from build123d import *

# Parameters (mm, degrees)
F1_DEPTH = 25
F2_R     = 3.99999


# Not quite as in the source:
# - a fillet or chamfer is up to 0.001 mm smaller than in the source, because OpenCascade refuses the exact size


with BuildPart() as f1:
    # F0 (on Top) → F1 (new body)
    with BuildSketch(Plane.XY):
        Polygon((18.5, 25), (18.5, -25), (26.5, -25), (26.5, 33), (18.5, 33), (-18.5, 33), (-26.5, 33), (-26.5, -25), (-18.5, -25), (-18.5, 25), align=None)
        Polygon((18.5, 33), (26.5, 33), (26.5, 49), (-26.5, 49), (-26.5, 33), (-18.5, 33), (-18.5, 41), (18.5, 41), align=None)
    extrude(amount=F1_DEPTH)

    # F2 (radius 4 in the source; OpenCascade refuses exactly that, so slightly less here)
    f2_edges = [f1.edges().sort_by_distance(p)[0] for p in [
        (-26.5, 49, 12.5),
        (26.5, 49, 12.5),
        (-18.5, -25, 12.5),
        (18.5, -25, 12.5),
        (-26.5, -25, 12.5),
        (26.5, -25, 12.5),
        (0, 33, 25),
        (-18.5, 37, 25),
        (0, 41, 25),
        (18.5, 37, 25),
        (-18.5, 0, 25),
        (0, 25, 25),
        (26.5, 12, 0),
        (26.5, 12, 25),
        (18.5, 0, 0),
        (22.5, -25, 0),
        (0, 49, 0),
        (-26.5, 12, 0),
        (-22.5, -25, 0),
        (-18.5, 0, 0),
        (0, 25, 0),
        (0, 33, 0),
        (-18.5, 37, 0),
        (0, 41, 0),
        (18.5, 37, 0),
        (18.5, 0, 25),
        (22.5, -25, 25),
        (0, 49, 25),
        (-26.5, 12, 25),
        (-22.5, -25, 25),
    ]]
    fillet(f2_edges, radius=F2_R)


solid = f1.part
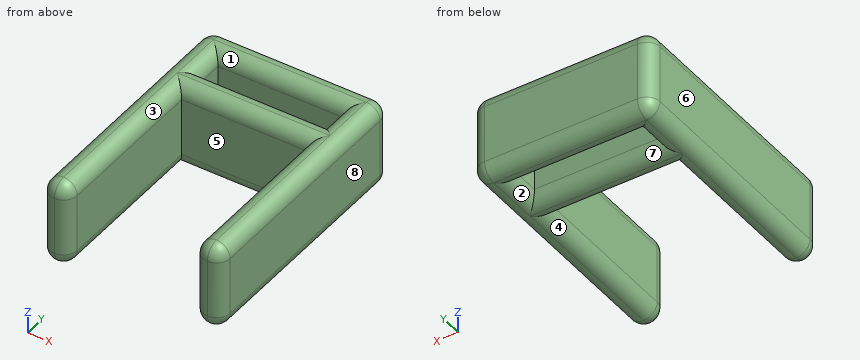
Here's how the part is built. I have some questions about the finished solid (model axes, mm). Face numbers are marked on the shaded views. A direction names the side the tool comes from. Coordinates: 2 decimals unless noted, no trailing zeros. Answer as CSV lines item,"result". Start each with the question number.
1. I need wall thicknesses on line 1 (Y direction, x = 14, z = 14.25); line 2 (X direction, y = 16.5, z = 9.5); line 3 (Y direction, x = -20, z = 9.75). Which ranges of each line are inside material? Lowest first, please. Write a range as [from, to].
2. On a 3-axis mill with a long thin cutter (end or side, diameter ignored), from which of +Z, -Z, +X, -X, +Y, -Y can I reach the whole of each face in a straight line? I mean the marked faces 1, 2, 3, 4 and 5. Say none if no direction works.
3. We'd pull the mould along X, two halves only. Please class the marked faces 6, 7 and 8: released by +X, released by -X, zero draft, split by the parting line, or undercut.
4. For pin 1 (6 mm diameter, centred on x = 12.5, z = 16.5, fed in from -Y); pin 2 (6 mm diameter, centred on y = 22, z = 3, fed in from +X); pin 3 (3 mm diameter, centred on x = -17.5, y = -4.5, fed in from +Z); pin 4 (5 mm diameter, centred on x = -10, y = 39.5, fed in from -Z), each with a flat end and sliding along its axis, tell me the tip position at first contact or that it passes through.
Recorded:
1,line 1,"y = [25, 33], [41, 49]"
1,line 2,"x = [-26.5, -18.5], [18.5, 26.5]"
1,line 3,"y = [-24.12, 49]"
2,face 1,"+Z"
2,face 2,"-Z"
2,face 3,"+Z, -Y"
2,face 4,"-Z, -Y"
2,face 5,"+Z, -Z, -Y"
3,face 6,"released by -X"
3,face 7,"undercut"
3,face 8,"released by +X"
4,pin 1,"stops at y = 25"
4,pin 2,"stops at x = 26.5"
4,pin 3,"stops at z = 22.94"
4,pin 4,"stops at z = 1.35"
